Model file for the job. Use its own axes, mm. Give positions to 0.01 mm unless a question says otherwise; leave off trailing zeros. Write each loop counter-clockwise with the first axis right and the second up, starting at its lowest first coordinate (ties: lowest second). Pieces come first, ordered by that corner, then holes.
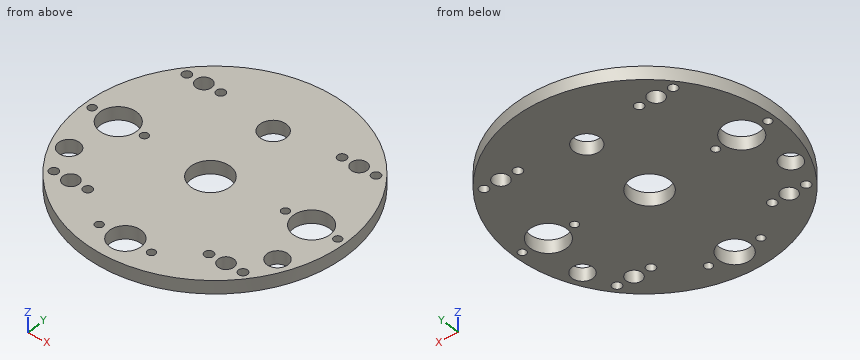
```python
from build123d import *

# Parameters (mm, degrees)
SKETCH1_R                  = 50
BOSS_EXTRUDE1_DEPTH        = 5
F_14_0_14_DIAMETER_HOLE1_D = 14
SKETCH7_R                  = 5
CUT_EXTRUDE1_DEPTH         = 10
SKETCH8_R                  = 3
CUT_EXTRUDE2_DEPTH         = 10
CIRPATTERN1_COUNT          = 4
SKETCH9_R                  = 7.5
CUT_EXTRUDE3_DEPTH         = 10
SKETCH10_R                 = 1.5
SKETCH10_R_2               = 6
CUT_EXTRUDE4_DEPTH         = 10
SKETCH12_R                 = 4
CUT_EXTRUDE5_DEPTH         = 10
M3_CLEARANCE_HOLE1_D       = 3.4
MIRROR3_COPY_1_D           = 3.4


with BuildPart() as part:
    # Sketch1 → Boss-Extrude1 (new body)
    with BuildSketch(Plane.XY):
        Circle(SKETCH1_R)
    extrude(amount=BOSS_EXTRUDE1_DEPTH)

    # Ø14.0 (14) Diameter Hole1 (through all)
    with Locations(Plane(origin=(0, 0, 0), x_dir=(-1, 0, 0), z_dir=(0, 0, -1))):
        with Locations((37, 0), (-37, 0)):
            Hole(F_14_0_14_DIAMETER_HOLE1_D / 2)

    # Sketch7 → Cut-Extrude1 (cut)
    with BuildSketch(Plane.XY.offset(5)):
        with Locations((0, 26)):
            Circle(SKETCH7_R)
    extrude(amount=-CUT_EXTRUDE1_DEPTH, mode=Mode.SUBTRACT)

    # Sketch8 → Cut-Extrude2 (cut)
    with BuildSketch(Plane.XY.offset(5)):
        with Locations((-29.69848481, 29.69848481)):
            Circle(SKETCH8_R)
    cut_extrude2 = extrude(amount=-CUT_EXTRUDE2_DEPTH, mode=Mode.SUBTRACT)

    # CirPattern1: Cut-Extrude2 ×4 about axis
    cirpattern1_axis = Axis((0, 0, 0), (0, 0, 1))
    for i in range(1, CIRPATTERN1_COUNT):
        add(cut_extrude2.rotate(cirpattern1_axis, i * 360 / CIRPATTERN1_COUNT), mode=Mode.SUBTRACT)

    # Sketch9 → Cut-Extrude3 (cut)
    with BuildSketch(Plane.XY.offset(5)):
        with Locations((0, -2)):
            Circle(SKETCH9_R)
    extrude(amount=-CUT_EXTRUDE3_DEPTH, mode=Mode.SUBTRACT)

    # Sketch10 → Cut-Extrude4 (cut)
    with BuildSketch(Plane.XY.offset(5)):
        with Locations((-47, 0)):
            Circle(SKETCH10_R)
        with Locations((-27, 0)):
            Circle(SKETCH10_R)
        with Locations((27, 0)):
            Circle(SKETCH10_R)
        with Locations((47, 0)):
            Circle(SKETCH10_R)
        with Locations((10, -40)):
            Circle(SKETCH10_R)
        with Locations((-10, -40)):
            Circle(SKETCH10_R)
        with Locations((0, -40)):
            Circle(SKETCH10_R_2)
    extrude(amount=-CUT_EXTRUDE4_DEPTH, mode=Mode.SUBTRACT)

    # Sketch12 → Cut-Extrude5 (cut)
    with BuildSketch(Plane.XY.offset(5)):
        with Locations((-39.87754263, -18.595203517)):
            Circle(SKETCH12_R)
    cut_extrude5 = extrude(amount=-CUT_EXTRUDE5_DEPTH, mode=Mode.SUBTRACT)

    # Mirror1: Cut-Extrude5 across plane
    add(cut_extrude5.mirror(Plane(origin=(0, 0, 0), x_dir=(0, 0, 1), z_dir=(1, 0, 0))), mode=Mode.SUBTRACT)

    # M3 Clearance Hole1 (through all)
    with Locations(Plane.XY.offset(5)):
        with Locations((-36.19848481, -29.69848481), (-23.19848481, -29.69848481)):
            m3_clearance_hole1 = Hole(M3_CLEARANCE_HOLE1_D / 2)

    # Mirror2: M3 Clearance Hole1 across plane
    add(m3_clearance_hole1.mirror(Plane.ZX), mode=Mode.SUBTRACT)

    # Mirror3: M3 Clearance Hole1 across plane
    add(m3_clearance_hole1.mirror(Plane(origin=(0, 0, 0), x_dir=(0, 0, 1), z_dir=(1, 0, 0))), mode=Mode.SUBTRACT)

    # Mirror3 copy 1 (through all)
    with Locations(Plane(origin=(0, 0, 5), x_dir=(-1, 0, 0), z_dir=(0, 0, 1))):
        with Locations((-36.19848481, -29.69848481), (-23.19848481, -29.69848481)):
            Hole(MIRROR3_COPY_1_D / 2)


solid = part.part
```
1. Probe probe 1 along Y at (x, z) = (-1.5, 1.35); probe 2 along Y at (x, z) = (-23, 4.5); probe 3 along X at (y, z) = (-16, 1.1). List the from-to ranges inside material, lowest first.
Calculated:
probe 1: y = -49.98 to -45.81, -34.19 to -9.35, 5.35 to 21.23, 30.77 to 49.98
probe 2: y = -44.4 to -31.39, -28.01 to 28.01, 31.39 to 44.4
probe 3: x = -47.37 to -42.92, -36.83 to 36.83, 42.92 to 47.37
2. Slice it at C-C, the plane x = 10. Write the cut outline in (y, z).
Calculated:
outline: (-48.99, 0) - (-41.5, 0) - (-41.5, 5) - (-48.99, 5) - close; (-38.5, 0) - (48.99, 0) - (48.99, 5) - (-38.5, 5) - close
3. Pin check, flat tips, straight feed: P1, Ø1.8, axis at x = 27, y = 0, coming from the -Z side; P2, Ø4, axis at x = -23.2, y = -29.7, coming from the -Z side; P3, Ø3, axis at y = -23.5, z = 2, coming from the +X side; P4, Ø2, axis at x = -13.5, z = 2.5, coming from the -Y side. Stop position of each tip, or through.
Calculated:
P1: passes through
P2: stops at z = 0
P3: stops at x = 44.9
P4: stops at y = -48.41
4. Slice it at B-B, the plane y = 0. State how many separate pieces and enclosed holes the cut face has, and give its area (3 significant figures).
Calculated:
separate pieces: 8
enclosed holes: 0
area: 228 mm2
5. Slice it at A-A, the plane x = 0. Write the cut outline in (y, z), and give its area (3 significant figures).
Calculated:
outline: (-50, 0) - (-46, 0) - (-46, 5) - (-50, 5) - close; (-34, 0) - (-9.5, 0) - (-9.5, 5) - (-34, 5) - close; (5.5, 0) - (21, 0) - (21, 5) - (5.5, 5) - close; (31, 0) - (50, 0) - (50, 5) - (31, 5) - close
area: 315 mm2
